Part model, mm, in its own coordinate system. Round coordinates to 2 decimals unless told otherwise and drop trailing zeros. Write each loop counter-clockwise with the first axis right and the second up, starting at its lowest first coordinate (ties: lowest second). Pieces come first, ordered by that corner, then holes. Notation, with made-up numbers: (-13, 67.25) -> (43, 67.25) arc R19 cw to (43, 78.25) -> close; hole circle Ø3 at (43.25, -14.5). An arc over 180 degrees is marked (long way). Use CSV: the item, a comma, the result in double quotes. Start each with the question number.
Autodesk Fusion 360 part; units mm, degrees
sketch "草图1" plane through (0, 0, 0) normal (0, 1, 0) x (1, 0, 0)
  line L0 (0, 0) -> (0, -25.7)
  line L1 (0, -25.7) -> (-4.625, -25.7)
  line L2 (-4.625, -25.7) -> (-4.625, -28)
  line L3 (-4.625, -28) -> (5.375, -28)
  line L4 (5.375, -28) -> (5.375, -25.7)
  line L5 (5.375, -25.7) -> (0.75, -25.7)
  line L6 (0.75, -25.7) -> (0.75, 0)
  line L7 (0.75, 0) -> (0, 0)
  line L8 (0.375, -28) -> (0.375, 0)
  line L9 (0.375, 0) -> (0.375, -0.4348)
  line L10 (0.375, 0) -> (0.75, -5)
  line L11 (0.375, 0) -> (0, -5)
  line L12 (0.75, -5) -> (0, -5)
  dimension "d1" = 2.3
  dimension "d2" = 0.75
  dimension "d3" = 5
  dimension "d4" = 28
  dimension "d5" = 10
extrude "拉伸1" add sketch "草图1" along normal blind 0.75 contours L0 L1 L2 L3 L8 L12 | L8 L9 L11 L12 | L8 L9 L10 L12 | L3 L4 L5 L6 L8 L12
fillet "圆角1" radius 1 4 edges at (5.375, 0.375, 28) (5.375, 0.375, 25.7) (-4.625, 0.375, 25.7) (-4.625, 0.375, 28)
fillet "圆角2" radius 0.375 18 edges at (-1.8125, 0, 25.7) (-4.3321, 0, 25.9929) (-4.625, 0, 26.85) (-4.3321, 0, 27.7071) (0.375, 0, 28) (5.0821, 0, 27.7071) (5.375, 0, 26.85) (5.0821, 0, 25.9929) (2.5625, 0, 25.7) (-1.8125, 0.75, 25.7) (-4.3321, 0.75, 25.9929) (-4.625, 0.75, 26.85) (-4.3321, 0.75, 27.7071) (0.375, 0.75, 28) (5.0821, 0.75, 27.7071) (5.375, 0.75, 26.85) (5.0821, 0.75, 25.9929) (2.5625, 0.75, 25.7)
fillet "圆角3" radius 0.325 8 edges at (0.75, 0, 15.5375) (0.75, 0.75, 15.5375) (0, 0.75, 15.5375) (0, 0, 15.5375) (0.5625, 0, 2.5) (0.5625, 0.75, 2.5) (0.1875, 0, 2.5) (0.1875, 0.75, 2.5)
sketch "草图2" plane through (0, 0, 0) normal (0, -1, 0) x (1, 0, 0)
  line L0 (0.425, 26.075) -> (4.375, 26.075)
  arc A0 (4.375, 26.075) -> (5, 26.7) centre (4.375, 26.7) ccw
  line L1 (5, 26.7) -> (5, 27)
  arc A1 (5, 27) -> (4.375, 27.625) centre (4.375, 27) ccw
  line L2 (4.375, 27.625) -> (-3.625, 27.625)
  arc A2 (-3.625, 27.625) -> (-4.25, 27) centre (-3.625, 27) ccw
  line L3 (-4.25, 27) -> (-4.25, 26.7)
  arc A3 (-4.25, 26.7) -> (-3.625, 26.075) centre (-3.625, 26.7) ccw
  line L4 (-3.625, 26.075) -> (0.325, 26.075)
  line L5 (0.325, 26.075) -> (0.325, 5.0122)
  line L6 (0.325, 5.0122) -> (0.375, 4.3455)
  line L7 (0.375, 4.3455) -> (0.425, 5.0122)
  line L8 (0.425, 5.0122) -> (0.425, 26.075)
  line L9 (-3.75, 27) -> (-3.75, 26.7)
  arc A4 (-3.75, 26.7) -> (-3.625, 26.575) centre (-3.625, 26.7) ccw
  line L10 (-3.625, 26.575) -> (-0.075, 26.575)
  line L11 (-0.075, 26.575) -> (0.825, 26.575)
  line L12 (0.825, 26.575) -> (4.375, 26.575)
  arc A5 (4.375, 26.575) -> (4.5, 26.7) centre (4.375, 26.7) ccw
  line L13 (4.5, 26.7) -> (4.5, 27)
  arc A6 (4.5, 27) -> (4.375, 27.125) centre (4.375, 27) ccw
  line L14 (4.375, 27.125) -> (-3.625, 27.125)
  arc A7 (-3.625, 27.125) -> (-3.75, 27) centre (-3.625, 27) ccw
  dimension "d14" = -0.5
extrude "拉伸2" cut sketch "草图2" against normal blind 3 contours L9 A4 L10 L11 L12 A5 L13 A6 L14 A7
equation "d11 = ( 0.75 / 2 ) * 1 mm"
1. Band-saw the part on B-B (z = 21.5). List the corners of the cut face in (x, y) (3 decimals).
2. Drill centre lines: line 1 along X through (y, z) = (0.45, 23.5); line 2 along Z through (x, y) = (3, 0.65) (3 decimals); line 3 along Z through (x, y) = (1, 0.3) (3 decimals). Where is each one in solid material? Low to high. Write a range as [from, to].
3. Band-saw the part on C-C (y = 0.15). List the corners of the cut face in (x, z) (3 decimals), then the cut area to 3 significant figures.
4. Flat gauge pin, fed straight in: pin 1 (1 mm diameter, centred on x = 3, z = 6, fed in from +Y). Where does the tip first touch, or does it go through?
Answers below:
1,outline,"(0, 0.325) arc R0.325 ccw to (0.325, 0) -> (0.425, 0) arc R0.325 ccw to (0.75, 0.325) -> (0.75, 0.425) arc R0.325 ccw to (0.425, 0.75) -> (0.325, 0.75) arc R0.325 ccw to (0, 0.425) -> close"
2,line 1,"x = [0, 0.75]"
2,line 2,"z = [25.82, 26.575], [27.125, 27.88]"
2,line 3,"z = [25.708, 26.575], [27.125, 27.992]"
3,outline,"(-4.55, 26.7) arc R0.925 ccw to (-3.625, 25.775) -> (0.051, 25.775) -> (0.051, 5) -> (0.375, 0.684) -> (0.699, 5.004) -> (0.699, 25.775) -> (4.375, 25.775) arc R0.925 ccw to (5.3, 26.7) -> (5.3, 27) arc R0.925 ccw to (4.375, 27.925) -> (-3.625, 27.925) arc R0.925 ccw to (-4.55, 27) -> close; hole (-3.75, 26.7) arc R0.125 ccw to (-3.625, 26.575) -> (4.375, 26.575) arc R0.125 ccw to (4.5, 26.7) -> (4.5, 27) arc R0.125 ccw to (4.375, 27.125) -> (-3.625, 27.125) arc R0.125 ccw to (-3.75, 27) -> close"
3,area,"30.8 mm^2"
4,pin 1,"passes through"
